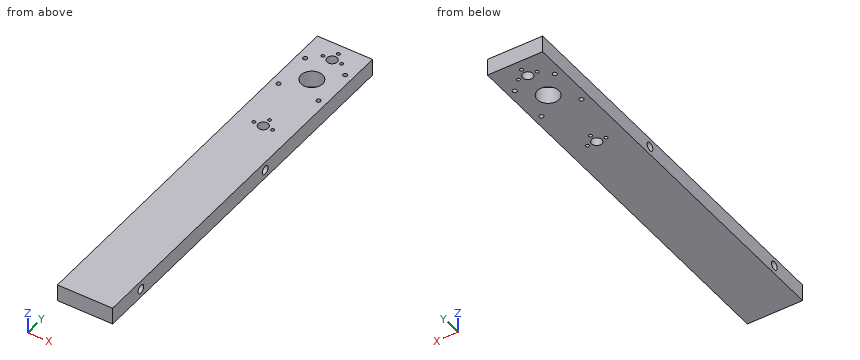
from build123d import *

# Parameters (mm, degrees)
SKETCH1_W           = 65
SKETCH1_H           = 460
SKETCH1_R           = 2.54
SKETCH1_R_2         = 6
SKETCH1_R_3         = 2
SKETCH1_R_4         = 12.7
BOSS_EXTRUDE1_DEPTH = 20
SKETCH2_R           = 5
CUT_EXTRUDE1_DEPTH  = 40


with BuildPart() as part:
    # Sketch1 → Boss-Extrude1 (new body)
    with BuildSketch(Plane.XY):
        with Locations((0, -191.425)):
            Rectangle(SKETCH1_W, SKETCH1_H)
        with Locations((-23.5712, 3.5712)):
            Circle(SKETCH1_R, mode=Mode.SUBTRACT)
        with Locations((23.5712, 3.5712)):
            Circle(SKETCH1_R, mode=Mode.SUBTRACT)
        with Locations((23.5712, -43.5712)):
            Circle(SKETCH1_R, mode=Mode.SUBTRACT)
        with Locations((-23.5712, -43.5712)):
            Circle(SKETCH1_R, mode=Mode.SUBTRACT)
        with Locations((0, -106)):
            Circle(SKETCH1_R_2, mode=Mode.SUBTRACT)
        with Locations((11, -106)):
            Circle(SKETCH1_R_3, mode=Mode.SUBTRACT)
        with Locations((0, -20)):
            Circle(SKETCH1_R_4, mode=Mode.SUBTRACT)
        with Locations((0, -95)):
            Circle(SKETCH1_R_3, mode=Mode.SUBTRACT)
        with Locations((0, 16)):
            Circle(SKETCH1_R_2, mode=Mode.SUBTRACT)
        with Locations((11, 16)):
            Circle(SKETCH1_R_3, mode=Mode.SUBTRACT)
        with Locations((-11, -106)):
            Circle(SKETCH1_R_3, mode=Mode.SUBTRACT)
        with Locations((0, 27)):
            Circle(SKETCH1_R_3, mode=Mode.SUBTRACT)
        with Locations((-11, 16)):
            Circle(SKETCH1_R_3, mode=Mode.SUBTRACT)
    extrude(amount=BOSS_EXTRUDE1_DEPTH)

    # Sketch2 → Cut-Extrude1 (cut, symmetric)
    with BuildSketch(Plane(origin=(0, 0, 0), x_dir=(0, 0, -1), z_dir=(1, 0, 0))):
        with Locations(Location((-10, -151.425, 0), (0, 0, 90))):
            Circle(SKETCH2_R)
        with Locations(Location((-10, -371.425, 0), (0, 0, 90))):
            Circle(SKETCH2_R)
    extrude(amount=CUT_EXTRUDE1_DEPTH, both=True, mode=Mode.SUBTRACT)


solid = part.part
Can you work these out from the model? Positions are in its coordinate system, mm. Give positions to 0.01 mm unless a question says otherwise; leave off trailing zeros. Write each loop counter-clockwise with the first axis right and the second up, starting at its lowest first coordinate (ties: lowest second). Pieces come first, ordered by that corner, then holes. Notation, with made-up numbers: M 35,59 L 87,59 A9 cw 87,65 Z; hole C -35,15.5 d2. An arc over 180 degrees is marked long. Answer in a Markdown table with one row per item. Add a question column.
Item 1: Imagine slicing it at A-A, the plane y = -20. Write out the boundary of the cut face in (x, z).
Item 2: For pin 1 Ø8 at (y, z) = (-151.425, 10) entering from -X, with a flat end and sliding along its axis, tell me the tip position at first contact or that it passes through.
Item 3: Please list where these lines run through material, in increasing order: L1, parallel to Y at x = -22, z = 9.75 (3 decimals); L2, parallel to Y at x = 11, z = 4 (3 decimals); L3, parallel to Y at x = 22, z = 11.75 (3 decimals).
Item 4: Imagine slicing it at B-B, the plane z = 10. State how many separate pieces and enclosed holes the cut face has, plus the area to 3 significant figures.
Evaluation:
| question | item | result |
|---|---|---|
| 1 | outline | M -32.5,0 L -12.7,0 L -12.7,20 L -32.5,20 Z; M 12.7,0 L 32.5,0 L 32.5,20 L 12.7,20 Z |
| 2 | pin 1 | passes through |
| 3 | L1 | y = -421.425 to -376.419, -366.431 to -156.419, -146.431 to -45.567, -41.575 to 1.575, 5.567 to 38.575 |
| 3 | L2 | y = -421.425 to -108, -104 to -26.347, -13.653 to 14, 18 to 38.575 |
| 3 | L3 | y = -421.425 to -376.109, -366.741 to -156.109, -146.741 to -45.567, -41.575 to 1.575, 5.567 to 38.575 |
| 4 | separate pieces | 3 |
| 4 | enclosed holes | 13 |
| 4 | area | 27,700 mm² |
